```python
from build123d import *

# Parameters (mm, degrees)
F0_W      = 1020
F0_H      = 730
F1_DEPTH  = 20
F2_W      = 20
F2_H      = 730
F3_DEPTH  = 580
F4_W      = 20
F4_H      = 730
F5_DEPTH  = 580
F6_W      = 980
F6_H      = 20
F7_DEPTH  = 580
F8_W      = 980
F8_H      = 20
F9_DEPTH  = 255
F10_W     = 100
F10_H     = 150
F11_DEPTH = 25


with BuildPart() as f1:
    # F0 (on Top) → F1 (new body)
    with BuildSketch(Plane.XY):
        with Locations((-510, 365)):
            Rectangle(F0_W, F0_H)
    extrude(amount=F1_DEPTH)

    # F2 (on face) → F3 (join)
    with BuildSketch(Plane.XY.offset(20)):
        with Locations((-10, 365)):
            Rectangle(F2_W, F2_H)
    extrude(amount=F3_DEPTH)

    # F4 (on face) → F5 (join)
    with BuildSketch(Plane.XY.offset(20)):
        with Locations((-1010, 365)):
            Rectangle(F4_W, F4_H)
    extrude(amount=F5_DEPTH)

    # F6 (on face) → F7 (join)
    with BuildSketch(Plane.XY.offset(20)):
        with Locations((-510, 461.57975)):
            Rectangle(F6_W, F6_H)
    extrude(amount=F7_DEPTH)

    # F8 (on face) → F9 (join)
    with BuildSketch(Plane(origin=(0, 471.57975, 0), x_dir=(-1, 0, 0), z_dir=(0, 1, 0))):
        with Locations((510, 361.820499)):
            Rectangle(F8_W, F8_H)
    extrude(amount=F9_DEPTH)

    # F10 (on face) → F11 (join)
    with BuildSketch(Plane(origin=(-20, 0, 0), x_dir=(0, -1, 0), z_dir=(-1, 0, 0))):
        with Locations((-521.57975, 95)):
            Rectangle(F10_W, F10_H)
    extrude(amount=F11_DEPTH)


solid = f1.part
```
Geometry check sheet. Reference: the model listing, model coordinates, mm. A direction names the side the tool comes from. Coordinates: 2 decimals unless noted, no trailing zeros. Order: outer loops, then holes, each group sorted by start corner. A loop starts at its lowest first (then second) coordinate and runs counter-clockwise, first axis right, second up.
Item 1: Section check A-A (z = 37). Enter the section's corners in (x, y).
Item 2: Section check C-C (x = -834). Enter the section's corners in (y, z).
Item 3: Section check D-D (y = 240.5). Enter the section's corners in (x, z).
Item 4: Tool access check on faces 1 (the flat face through (-503, 597, 371.82)), 2 (the flat face through (-1000, 223, 306)), 3 (the flat face through (-45, 522, 96)). Record the directions out of +Z, -Z, +X, -X, +Y, -Y that give a thin tool (end or side, any length) a straight path to the whole face; none if there is none.
Item 5: Scan lines: line 1 along X through (y, z) = (663, 382); line 2 along Z through (x, y) = (-353, 664); line 3 along Y through (x, z) = (-313.5, 372.5). Record each from-to range of solid material in increasing order.
Item 6: Section check B-B (y = 588.5). Enter the section's corners in (x, z).
Item 7: Mould release check, pull along X, two halves, no side actions. Record for faces 4 (the flat face through (-517, 229, 20)), 5 (the flat face through (-1020, 360, 296)), 6 (the flat face through (0, 360, 296)), 7 (the flat face through (-739, 0, 10)): released by +X, released by -X, zero draft, split by the parting line, or undercut.
Item 8: Depth check by flat-ended pin: pin 1 (8 mm diameter, centred on x = -169.5, y = 124, fed in from +Z); pin 2 (12 mm diameter, centred on x = -811.5, y = 116, fed in from -Z); pin 3 (10 mm diameter, centred on x = -450, z = 406.5, fed in from +Y); pin 4 (1 mm diameter, centred on x = -704.5, z = 302, fed in from -Y). Enter the tip coordinate at first touch or a pass-through.
Check sheet entries:
1. outline: (-1020, 0) - (-1000, 0) - (-1000, 451.58) - (-20, 451.58) - (-20, 0) - (0, 0) - (0, 730) - (-20, 730) - (-20, 571.58) - (-45, 571.58) - (-45, 471.58) - (-1000, 471.58) - (-1000, 730) - (-1020, 730) - close
2. outline: (0, 0) - (730, 0) - (730, 20) - (471.58, 20) - (471.58, 351.82) - (726.58, 351.82) - (726.58, 371.82) - (471.58, 371.82) - (471.58, 600) - (451.58, 600) - (451.58, 20) - (0, 20) - close
3. outline: (-1020, 0) - (0, 0) - (0, 600) - (-20, 600) - (-20, 20) - (-1000, 20) - (-1000, 600) - (-1020, 600) - close
4. face 1: +Z, +Y
4. face 2: +Z, -Y
4. face 3: +Y
5. line 1: x = -1020 to -1000, -20 to 0
5. line 2: z = 0 to 20, 351.82 to 371.82
5. line 3: y = 451.58 to 471.58
6. outline: (-1020, 0) - (0, 0) - (0, 600) - (-20, 600) - (-20, 371.82) - (-1000, 371.82) - (-1000, 600) - (-1020, 600) - close; hole (-1000, 20) - (-20, 20) - (-20, 351.82) - (-1000, 351.82) - close
7. face 4: undercut
7. face 5: released by -X
7. face 6: released by +X
7. face 7: zero draft
8. pin 1: stops at z = 20
8. pin 2: stops at z = 0
8. pin 3: stops at y = 471.58
8. pin 4: stops at y = 451.58
